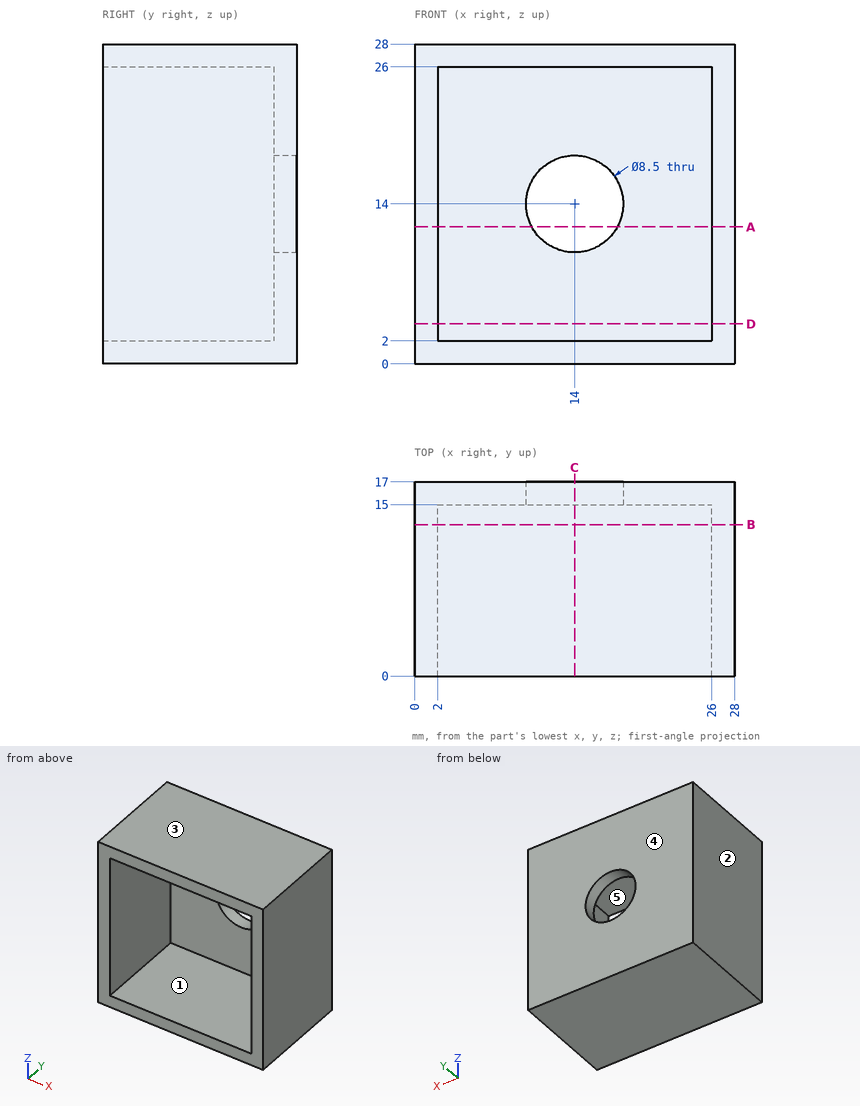
Check sheet for the drawn part. Datum: minimum x, y, z corner. Units: mm. A direction names the side the tool comes from. Round coordinates to 2 decimals unless told otherwise and drop trailing zeros. Loops run counter-clockwise (first coordinate to the right, second up) from the corner with the lowest first, then second, coordinate; pieces in that order, holes last. Notation, with made-up numbers: (29, -17) - (37, -17) arc R28 ccw to (37, 5) - close; hole circle Ø7 at (-30.5, 87.5). An arc over 180 degrees is marked (long way). Answer as a JSON object with one key per item and string values. Group by question number.
Q1. Sectioned sample at D-D, the plane z = 3.5. Enter the section's corners in (x, y).
Q2. Mould release check, pull along Z, two halves, no side actions. Record for the marked faces 1, 2 and 3: released by +Z, released by -Z, zero draft, split by the parting line, or undercut.
Q3. Sectioned sample at B-B, the plane y = 13.25. Enter the section's corners in (x, z).
Q4. Sectioned sample at C-C, the plane x = 14. Enter the section's corners in (y, z).
Q5. Set-up check for the marked faces 4 and 5: record each of +Z, -Z, +X, -X, +Y, -Y from which the full face is reachable in a straight line by a thin tool's end or side.
Q6. Gauge pin test, flat end, axial feed: P1, Ø13.5, axis at x = 14, z = 14, coming from the -Y side. Record the tip position at first contact, or that the pin passes through.
Q7. Sectioned sample at A-A, the plane z = 12. Enter the section's corners in (x, y), plus the area to 3 significant figures.
Q8. Scan lines: line 1 along Z through (x, y) = (15.5, 10.75); line 2 along X through (y, z) = (15.95, 14). Record each from-to range of solid material in increasing order. Write a range as [from, to].
Solution:
{
 "1": {"outline": "(0, 0) - (2, 0) - (2, 15) - (26, 15) - (26, 0) - (28, 0) - (28, 17) - (0, 17) - close"},
 "2": {"face 1": "undercut", "face 2": "zero draft", "face 3": "released by +Z"},
 "3": {"outline": "(0, 0) - (28, 0) - (28, 28) - (0, 28) - close; hole (2, 2) - (26, 2) - (26, 26) - (2, 26) - close"},
 "4": {"outline": "(0, 0) - (17, 0) - (17, 9.75) - (15, 9.75) - (15, 2) - (0, 2) - close; (0, 26) - (15, 26) - (15, 18.25) - (17, 18.25) - (17, 28) - (0, 28) - close"},
 "5": {"face 4": "+Z, -Z, +X, -X, +Y", "face 5": "-Y"},
 "6": {"P1": "stops at y = 15"},
 "7": {"outline": "(0, 0) - (2, 0) - (2, 15) - (10.25, 15) - (10.25, 17) - (0, 17) - close; (17.75, 15) - (26, 15) - (26, 0) - (28, 0) - (28, 17) - (17.75, 17) - close", "area": "101 mm²"},
 "8": {"line 1": "z = [0, 2], [26, 28]", "line 2": "x = [0, 9.75], [18.25, 28]"}
}
